Could you check a few things on this model? Use its own coordinates, in mm. Give positions to 0.01 mm unless a question says otherwise; leave off trailing zeros. Loops run counter-clockwise (first coordinate to the right, second up) from the corner with the lowest first, then second, coordinate; pieces in that order, holes last. Notation, with made-up numbers: M 51.25,25.25 L 88.25,25.25 A10 cw 88.25,31.25 Z; hole C -2.75,25 d5. An arc over 180 degrees is marked long. Answer in a Markdown table with one row per item. Add a question column.
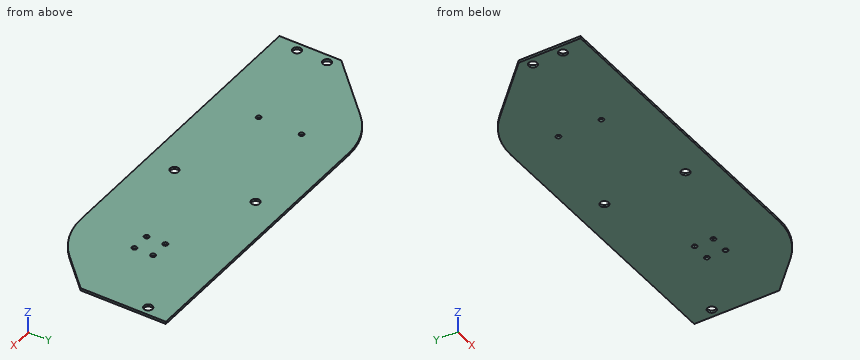
```python
from build123d import *

# Parameters (mm, degrees)
F0_R     = 3.175
F0_R_2   = 1.8288
F1_DEPTH = 1.778


with BuildPart() as f1:
    # F0 (on Top) → F1 (new body)
    with BuildSketch(Plane.XY):
        with BuildLine():
            Line((133.35, -12.1520489686), (133.35, 50.8))
            Line((133.35, 50.8), (73.66, 50.8))
            ThreePointArc((73.66, 50.8), (109.5810244843, 35.9210244843), (124.46, 0))
            ThreePointArc((124.46, 0), (120.5930802516, -19.4403183641), (109.5810244843, -35.9210244843))
            Line((109.5810244843, -35.9210244843), (133.35, -12.1520489686))
        make_face()
        with Locations((127, 33.655)):
            Circle(F0_R, mode=Mode.SUBTRACT)
        with BuildLine():
            ThreePointArc((73.66, -50.8), (22.86, 0), (73.66, 50.8))
            Line((73.66, 50.8), (-73.6599997452, 50.8))
            ThreePointArc((-73.6599997452, 50.8), (-37.7389754256, 35.9210243942), (-22.86, 0))
            ThreePointArc((-22.86, 0), (-37.7389756058, -35.9210245744), (-73.6600002548, -50.8))
            Line((-73.6600002548, -50.8), (73.66, -50.8))
        make_face()
        with Locations((0, -29.972)):
            Circle(F0_R, mode=Mode.SUBTRACT)
        with Locations((0, 29.972)):
            Circle(F0_R, mode=Mode.SUBTRACT)
        with BuildLine():
            ThreePointArc((124.46, 0), (109.5810244843, 35.9210244843), (73.66, 50.8))
            ThreePointArc((73.66, 50.8), (22.86, 0), (73.66, -50.8))
            ThreePointArc((73.66, -50.8), (93.1003183641, -46.9330802516), (109.5810244843, -35.9210244843))
            ThreePointArc((109.5810244843, -35.9210244843), (120.5930802516, -19.4403183641), (124.46, 0))
        make_face()
        with Locations((66.7452027868, -6.9147972132)):
            Circle(F0_R_2, mode=Mode.SUBTRACT)
        with Locations((80.5747972132, -6.9147972132)):
            Circle(F0_R_2, mode=Mode.SUBTRACT)
        with Locations((66.7452027868, 6.9147972132)):
            Circle(F0_R_2, mode=Mode.SUBTRACT)
        with Locations((80.5747972132, 6.9147972132)):
            Circle(F0_R_2, mode=Mode.SUBTRACT)
        with BuildLine():
            ThreePointArc((-22.86, 0), (-37.7389754256, 35.9210243942), (-73.6599997452, 50.8))
            ThreePointArc((-73.6599997452, 50.8), (-93.1003182465, 46.9330803003), (-109.5810244843, 35.9210244843))
            ThreePointArc((-109.5810244843, 35.9210244843), (-120.5930803003, -19.4403182465), (-73.6600002548, -50.8))
            ThreePointArc((-73.6600002548, -50.8), (-37.7389756058, -35.9210245744), (-22.86, 0))
        make_face()
        with Locations((-73.66, -15.875)):
            Circle(F0_R_2, mode=Mode.SUBTRACT)
        with Locations((-73.66, 15.875)):
            Circle(F0_R_2, mode=Mode.SUBTRACT)
        with BuildLine():
            ThreePointArc((-73.6600002548, -50.8), (-120.5930803003, -19.4403182465), (-109.5810244843, 35.9210244843))
            Line((-109.5810244843, 35.9210244843), (-133.35, 12.1520489686))
            Line((-133.35, 12.1520489686), (-133.35, -50.8))
            Line((-133.35, -50.8), (-73.6600002548, -50.8))
        make_face()
        Polygon((-133.35, -50.8), (-133.35, 12.1520489686), (-150.5712, -5.0691510314), (-150.5712, -50.8), align=None)
        with Locations((-144.2212, -33.655)):
            Circle(F0_R, mode=Mode.SUBTRACT)
        with Locations((-144.2212, -11.43)):
            Circle(F0_R, mode=Mode.SUBTRACT)
    extrude(amount=F1_DEPTH)


solid = f1.part
```
Item 1: Suppose I cut it at A-A (x = 0). List the corners of the cut face in (y, z) for me.
Item 2: Suppose I cut it at C-C (y = 1). List the corners of the cut face in (x, z) for me.
Item 3: I need wall thicknesses on L1, parallel to Y at x = 0, z = 0.55; L2, parallel to Y at x = 1.5, z = 1; L3, parallel to X at y = -8, z = 0.8. Which ranges of each line are inside material? Lowest first, please.
Item 4: Suppose I cut it at B-B (z = 0.3). Give the number of separate pieces and of enclosed holes in the cut face, then the cut area to 3 significant figures.
Item 5: Suppose I cut it at D-D (x = -99). List the corners of the cut face in (y, z) for me, then the cut area to 3 significant figures.
Values found:
| question | item | result |
|---|---|---|
| 1 | outline | M -50.8,0 L -33.15,0 L -33.15,1.78 L -50.8,1.78 Z; M -26.8,0 L 26.8,0 L 26.8,1.78 L -26.8,1.78 Z; M 33.15,0 L 50.8,0 L 50.8,1.78 L 33.15,1.78 Z |
| 2 | outline | M -144.5,0 L 133.35,0 L 133.35,1.78 L -144.5,1.78 Z |
| 3 | L1 | -50.8 to -33.15, -26.8 to 26.8, 33.15 to 50.8 |
| 3 | L2 | -50.8 to -32.77, -27.17 to 27.17, 32.77 to 50.8 |
| 3 | L3 | -150.57 to 65.27, 68.22 to 79.1, 82.05 to 133.35 |
| 4 | separate pieces | 1 |
| 4 | enclosed holes | 11 |
| 4 | area | 26,200 mm² |
| 5 | outline | M -50.8,0 L 44.03,0 L 44.03,1.78 L -50.8,1.78 Z |
| 5 | area | 169 mm² |
